CAD build for the part. Positions are in the model's coordinates, mm. Face numbers are marked on the shaded views. A direction names the side the tool comes from. Give positions to 0.01 mm unless a question says otherwise; leave off trailing zeros. Write each loop counter-clockwise with the first axis right and the second up, starting at its lowest first coordinate (ties: lowest second). Pieces come first, ordered by that corner, then holes. Notation, with made-up numbers: (-31, 11.25) - (26, 11.25) arc R12 cw to (26, 27.25) - close; hole circle Ø2 at (59, -34). An arc over 180 degrees is marked (long way). Answer as a JSON object with one key per item and string values.
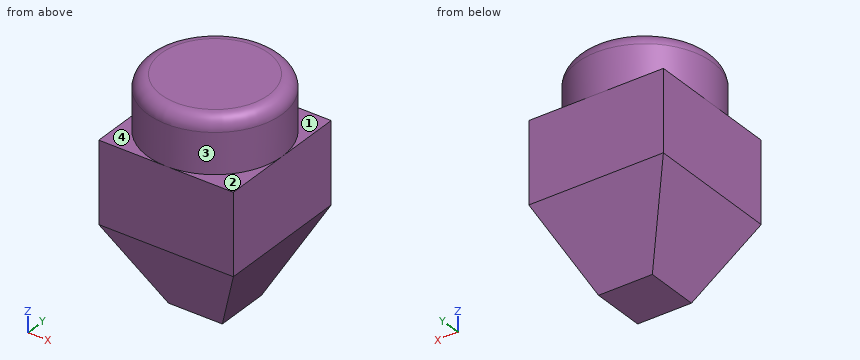
from build123d import *
from OCP.BRepFilletAPI import BRepFilletAPI_MakeChamfer

# Parameters (mm, degrees)
SCHIZZO1_R                   = 5
ESTRUSIONE_ESTRUSIONE1_DEPTH = 4
SCHIZZO2_W                   = 10
SCHIZZO2_H                   = 10
ESTRUSIONE_ESTRUSIONE2_DEPTH = 12
RACCORDO1_R                  = 1
SMUSSO1_SIZE                 = 6
SMUSSO1_SIZE2                = 3


with BuildPart() as part:
    # Schizzo1 → Estrusione-Estrusione1 (new body)
    with BuildSketch(Plane.XY):
        Circle(SCHIZZO1_R)
    extrude(amount=ESTRUSIONE_ESTRUSIONE1_DEPTH)

    # Schizzo2 → Estrusione-Estrusione2 (add)
    with BuildSketch(Plane(origin=(0, 0, 0), x_dir=(-1, 0, 0), z_dir=(0, 0, -1))):
        Rectangle(SCHIZZO2_W, SCHIZZO2_H)
    extrude(amount=ESTRUSIONE_ESTRUSIONE2_DEPTH)

    # Raccordo1
    raccordo1_edges = [part.edges().sort_by_distance(p)[0] for p in [
        (-5, 0, 4),
    ]]
    fillet(raccordo1_edges, radius=RACCORDO1_R)

    # Smusso1: one chamfer whose edges measure the first distance from different faces: ONE call of the kernel's chamfer builder (chamfer() names one face for all edges)
    smusso1_edges_1 = [part.edges().sort_by_distance(p)[0] for p in [
        (0, 5, -12),
    ]]
    smusso1_side_1 = [part.faces().sort_by_distance(p)[0] for p in [
        (0, 5, -6),
    ]]
    smusso1_edges_2 = [part.edges().sort_by_distance(p)[0] for p in [
        (5, 0, -12),
    ]]
    smusso1_side_2 = [part.faces().sort_by_distance(p)[0] for p in [
        (5, 0, -6),
    ]]
    smusso1_edges_3 = [part.edges().sort_by_distance(p)[0] for p in [
        (0, -5, -12),
    ]]
    smusso1_side_3 = [part.faces().sort_by_distance(p)[0] for p in [
        (0, -5, -6),
    ]]
    smusso1_edges_4 = [part.edges().sort_by_distance(p)[0] for p in [
        (-5, 0, -12),
    ]]
    smusso1_side_4 = [part.faces().sort_by_distance(p)[0] for p in [
        (-5, 0, -6),
    ]]
    smusso1 = BRepFilletAPI_MakeChamfer(part.part.solid().wrapped)
    for e in smusso1_edges_1:
        smusso1.Add(SMUSSO1_SIZE, SMUSSO1_SIZE2, e.wrapped, smusso1_side_1[0].wrapped)  # the first distance lies on this face
    for e in smusso1_edges_2:
        smusso1.Add(SMUSSO1_SIZE, SMUSSO1_SIZE2, e.wrapped, smusso1_side_2[0].wrapped)  # the first distance lies on this face
    for e in smusso1_edges_3:
        smusso1.Add(SMUSSO1_SIZE, SMUSSO1_SIZE2, e.wrapped, smusso1_side_3[0].wrapped)  # the first distance lies on this face
    for e in smusso1_edges_4:
        smusso1.Add(SMUSSO1_SIZE, SMUSSO1_SIZE2, e.wrapped, smusso1_side_4[0].wrapped)  # the first distance lies on this face
    add(Compound.cast(smusso1.Shape()), mode=Mode.REPLACE)


solid = part.part
Item 1: Probe line 1 (Y direction, x = 1.5, z = 2.75); line 2 (X direction, y = -3, z = -9.5); line 3 (Z direction, x = -3.25, y = -0.25). List the from-to ranges inside material, lowest first. Write a range as from..to.
Entries:
{"line 1": "-4.77..4.77", "line 2": "-3.25..3.25", "line 3": "-9.5..4"}
Item 2: Flat gauge pin, fed straight in: P1, Ø1.5, axis at x = 4, y = 2, coming from the -Z side. Where does the tip first touch, or does it go through?
Entries:
{"P1": "z = -9.5"}
Item 3: Which spindle directions (+Z, -Z, +X, -X, +Y, -Y) get a long thin tool onto all of the face, cutting with end or side? Do the marked faces 1, 2, 3 and 4. Say none if no direction does.
Entries:
{"face 1": "+Z, +X, +Y", "face 2": "+Z, +X, -Y", "face 3": "+Z", "face 4": "+Z, -X, -Y"}
Item 4: Cut at A-A (z = -7.75). Give the cut face in (x, y) (3 decimals), and give its area (3 significant figures).
Entries:
{"outline": "(-4.125, -4.125) - (4.125, -4.125) - (4.125, 4.125) - (-4.125, 4.125) - close", "area": "68.1 mm2"}
